```python
from build123d import *

# Parameters (mm, degrees)
F0_W     = 88.9
F0_H     = 88.9
F1_DEPTH = 5.08
F2_DEPTH = 6.35
F3_DEPTH = 6.35
F5_ANGLE = -30
F6_D     = 2


with BuildPart() as f1:
    # F0 (on Top) → F1 (new body)
    with BuildSketch(Plane.XY):
        Rectangle(F0_W, F0_H)
        with BuildLine():
            ThreePointArc((0, 38.1), (26.940768, 26.940768), (38.1, 0))
            ThreePointArc((38.1, 0), (26.940768, -26.940768), (0, -38.1))
            ThreePointArc((0, -38.1), (-38.1, 0), (0, 38.1))
        make_face(mode=Mode.SUBTRACT)
    extrude(amount=F1_DEPTH)

    # F0 (on Top) → F2 (join)
    with BuildSketch(Plane.XY):
        with BuildLine():
            Line((0, 34.925), (0, 38.1))
            ThreePointArc((0, 38.1), (-38.1, 0), (0, -38.1))
            Line((0, -38.1), (0, -34.925))
            ThreePointArc((0, -34.925), (-34.925, 0), (0, 34.925))
        make_face()
    extrude(amount=F2_DEPTH)

    # F0 (on Top) → F3 (join)
    with BuildSketch(Plane.XY):
        with BuildLine():
            ThreePointArc((0, -38.1), (26.940768, -26.940768), (38.1, 0))
            ThreePointArc((38.1, 0), (26.940768, 26.940768), (0, 38.1))
            Line((0, 38.1), (0, 34.925))
            ThreePointArc((0, 34.925), (24.695704, 24.695704), (34.925, 0))
            ThreePointArc((34.925, 0), (24.695704, -24.695704), (0, -34.925))
            Line((0, -34.925), (0, -38.1))
        make_face()
    extrude(amount=F3_DEPTH)

    # F4 (on face) → F5 (revolve)
    with BuildSketch(Plane.XY.offset(6.35)):
        with BuildLine():
            Line((0, -38.1), (0, -34.925))
            ThreePointArc((0, -34.925), (-34.925, 0), (0, 34.925))
            Line((0, 34.925), (0, 38.1))
            ThreePointArc((0, 38.1), (-38.1, 0), (0, -38.1))
        make_face()
    revolve(axis=Axis((0, -36.5125, 6.35), (0, -1, 0)), revolution_arc=F5_ANGLE)

    # F6 (through all)
    with Locations(Plane(origin=(0, 0, 0), x_dir=(1, 0, 0), z_dir=(0, 0, -1))):
        with Locations((35.56, 35.56), (35.56, -35.56), (-35.56, -35.56), (-35.56, 35.56)):
            Hole(F6_D / 2)


solid = f1.part
```
Here's how the part is built. I have some questions about the finished solid (model axes, mm). A direction names the side the tool comes from. Give positions to 0.01 mm unless a question says otherwise; leave off trailing zeros. Loops run counter-clockwise (first coordinate to the right, second up) from the corner with the lowest first, then second, coordinate; pieces in that order, holes last. Notation, with made-up numbers: M 41.5,50.5 L 58.5,50.5 A9 cw 58.5,60.5 Z; hole C 33.25,-33 d5. An arc over 180 degrees is marked long. Return JSON: item names as keys, results as strings.
Item 1: I'm going to push flat-ended pins straight in: pin 1 Ø1.5 at (y, z) = (-23, 8.5) entering from -X; pin 2 Ø1.5 at (x, y) = (5, -34.5) entering from +Z; pin 3 Ø1.2 at (x, y) = (35.56, 35.56) entering from -Z; pin 4 Ø1.5 at (y, z) = (-23.5, 7) entering from +X. Where does each tip first touch, or does it pass through?
A:
{"pin 1": "stops at x = -30.86", "pin 2": "stops at z = 6.35", "pin 3": "passes through", "pin 4": "stops at x = 30.28"}
Item 2: Imagine slicing it at B-B on x = 27. List the corners of the cut face in (y, z) for me, then the cut area to 3 significant figures.
A:
{"outline": "M -44.45,0 L -22.15,0 L -22.15,6.35 L -26.88,6.35 L -26.88,5.08 L -44.45,5.08 Z; M 22.15,0 L 44.45,0 L 44.45,5.08 L 26.88,5.08 L 26.88,6.35 L 22.15,6.35 Z", "area": "239 mm^2"}
Item 3: Imagine slicing it at A-A on z = 3.75. List the corners of the cut face in (x, y) for me (3 decimals).
A:
{"outline": "M -44.45,-44.45 L 44.45,-44.45 L 44.45,44.45 L -44.45,44.45 Z; hole C -35.56,-35.56 d2; hole C -35.56,35.56 d2; hole M 0,-34.925 A34.925 ccw 34.925,0 A34.925 ccw 0,34.925 A34.925 ccw Z; hole C 35.56,-35.56 d2; hole C 35.56,35.56 d2"}
Item 4: On a 3-axis mill with a long thin cutter (end or side, diameter ignored), from which of +Z, -Z, +X, -X, +Y, -Y can I reach the whole of each face in a straight line? I mean faces 4 (the flat face through (39, 1, 5.08)), 5 (the flat face through (36, 0, 6.35)), 6 (the cylindrical face through (34.606, -35.86, 2.576)). Say none if no direction works.
A:
{"face 4": "+Z", "face 5": "+Z, +X, +Y, -Y", "face 6": "+Z, -Z"}
Item 5: Imagine slicing it at C-C on y = -27. List the corners of the cut face in (x, z) for me.
A:
{"outline": "M -44.45,0 L -22.15,0 L -22.15,6.35 A22.15 cw -19.19,17.43 L -23.28,19.79 A26.88 ccw -26.88,6.35 L -26.88,5.08 L -44.45,5.08 Z; M 22.15,0 L 44.45,0 L 44.45,5.08 L 26.88,5.08 L 26.88,6.35 L 22.15,6.35 Z"}
Item 6: Imagine slicing it at D-D on z = 9. List the corners of the cut face in (x, y) for me, then the cut area to 3 significant figures.
A:
{"outline": "M -4.59,-37.73 L -4.59,-34.52 A34.82 cw -4.59,34.52 L -4.59,37.73 A38.01 ccw Z", "area": "335 mm^2"}
Item 7: Thinking about a two-plate mould opening in X: for faces 1 (the flat face through (-1, -44.45, 3)), 2 (the flat face through (-44.45, -1, 3)), 3 (the cylindrical face through (-36.1, 34.72, 2.58)), which applies, released by +X, released by -X, zero draft, split by the parting line, or undercut?
A:
{"face 1": "zero draft", "face 2": "released by -X", "face 3": "undercut"}
Item 8: Please list where these lines run through material, in increasing order: line 1 (X direction, y = 35.56, z = 3.55); line 2 (Z direction, x = -40.5, y = 19).
A:
{"line 1": "x = -44.45 to -36.56, -34.56 to 34.56, 36.56 to 44.45", "line 2": "z = 0 to 5.08"}
